Verification items for the finished model (mm, model axes). Give positions to 0.01 mm unless a question says otherwise; leave off trailing zeros. Order: outer loops, then holes, each group sorted by start corner. A loop starts at its lowest first (then second) coordinate and runs counter-clockwise, first axis right, second up. Notation, with made-up numbers: M 22,76 L 74,76 A11 cw 74,90 Z; hole C 79,42.25 d1. An arc over 180 degrees is marked long. Answer as a JSON object with one key per item and string values.
```python
from build123d import *

# Parameters (mm, degrees)
F0_W     = 2200
F0_H     = 400
F1_DEPTH = 25
F2_R     = 10
F3_DEPTH = 25
F4_R     = 10
F5_DEPTH = 25
F6_DEPTH = 100
F7_DEPTH = 100
F8_SIZE  = 24.99999


# Not quite as in the source:
# - a fillet or chamfer is up to 0.001 mm smaller than in the source, because OpenCascade refuses the exact size


with BuildPart() as f1:
    # F0 (on Front) → F1 (new body)
    with BuildSketch(Plane.XZ):
        Rectangle(F0_W, F0_H)
    extrude(amount=F1_DEPTH)

    # F2 (on face) → F3 (cut)
    with BuildSketch(Plane.XZ.offset(25)):
        with Locations((977.5, -77.5)):
            Circle(F2_R)
    extrude(amount=-F3_DEPTH, mode=Mode.SUBTRACT)

    # F4 (on face) → F5 (cut)
    with BuildSketch(Plane.XZ.offset(25)):
        with Locations((-977.5, -77.5)):
            Circle(F4_R)
    extrude(amount=-F5_DEPTH, mode=Mode.SUBTRACT)

    # F6 (add): a face of the model
    f6_faces = [f1.faces().sort_by_distance(p)[0] for p in [
        (0, -12.5, 200),
    ]]
    extrude(f6_faces, amount=F6_DEPTH)

    # F7 (cut): a face of the model
    f7_faces = [f1.faces().sort_by_distance(p)[0] for p in [
        (0, -12.5, -200),
    ]]
    extrude(f7_faces, amount=-F7_DEPTH, mode=Mode.SUBTRACT)

    # F8 (size 25 in the source; OpenCascade refuses exactly that, so slightly less here)
    f8_edges = [f1.edges().sort_by_distance(p)[0] for p in [
        (-1100, -25, 100),
        (0, -25, 300),
        (1100, -25, 100),
    ]]
    chamfer(f8_edges, length=F8_SIZE)


solid = f1.part
```
Q1. Material ranges on L1, parallel to Z at x = -977.5, y = -6.5; L2, parallel to Z at x = 977.5, y = -14; L3, parallel to X at y = -22.5, z = 15.5, recorded low to high.
Resolved:
{"L1": "z = -100 to -87.5, -67.5 to 293.5", "L2": "z = -100 to -87.5, -67.5 to 286", "L3": "x = -1077.5 to 1077.5"}
Q2. Section check A-A on y = -13. Record the cut outline in (x, z), then the cut area to 3 significant figures.
Resolved:
{"outline": "M -1087,-100 L 1087,-100 L 1087,287 L -1087,287 Z; hole C -977.5,-77.5 d20; hole C 977.5,-77.5 d20", "area": "841,000 mm²"}
Q3. Gauge pin test, flat ends, axial feed: pin 1 Ø12 at (x, y) = (540.5, -13) entering from +Z; pin 2 Ø8 at (y, z) = (-14, 174.5) entering from -X; pin 3 Ø6 at (x, y) = (873, -20.5) entering from +Z. Record the tip position at first contact, or that the pin passes through.
Resolved:
{"pin 1": "stops at z = 293", "pin 2": "stops at x = -1090", "pin 3": "stops at z = 282.5"}
